from build123d import *

# Parameters (mm, degrees)
ESQUISSE5_W        = 4.75
ESQUISSE5_H        = 4.75
BOSS_EXTRU_3_DEPTH = 4
BOSS_EXTRU_4_DEPTH = 4


with BuildPart() as part:
    # Esquisse1 → Révolution1 (revolve)
    with BuildSketch(Plane(origin=(0, 0, 0), x_dir=(1, 0, 0), z_dir=(0, 1, 0))):
        Polygon((0, 0), (0, 4.75), (142, 4.75), (142, 0), (125.25, 0), (117.25, 0), (24.75, 0), (16.75, 0), align=None)
    revolve(axis=Axis((0, 0, -4.75), (1, 0, 0)))

    # Esquisse5 → Boss.-Extru.3 (add)
    with BuildSketch(Plane(origin=(142, 0, 0), x_dir=(0, 0, -1), z_dir=(1, 0, 0))):
        with Locations((4.75, 0)):
            Rectangle(ESQUISSE5_W, ESQUISSE5_H)
    extrude(amount=BOSS_EXTRU_3_DEPTH)

    # Esquisse6 → Boss.-Extru.4 (add)
    with BuildSketch(Plane.ZY):
        Polygon((-4.75, 2.375), (-7.125, 2.375), (-7.125, -2.375), (-2.375, -2.375), (-2.375, 2.375), align=None)
    extrude(amount=BOSS_EXTRU_4_DEPTH)


solid = part.part
CAD build for the part. Positions are in the model's coordinates, mm. A direction names the side the tool comes from. Coordinates: 2 decimals unless noted, no trailing zeros. Loops run counter-clockwise (first coordinate to the right, second up) from the corner with the lowest first, then second, coordinate; pieces in that order, holes last. Notation, with made-up numbers: (89, 62) - (140, 62) arc R21 ccw to (140, 78) - close; hole circle Ø2 at (-35, -38.75). An arc over 180 degrees is marked (long way). Use one line per item in the form item = value. Start each with the question number.
1) Tool access for faces 1 (the face through (144, 0, -7.125)), 2 (the face through (-2, 0, -7.125)), 3 (the face through (-2, 0, -2.375)): list every direction of +Z, -Z, +X, -X, +Y, -Y with a clear straight run to the whole face (end or side of a thin tool).
2) Band-saw the part on A-A (z = -4.75). Give the cut face in (x, y) (3 decimals), and give its area (3 significant figures).
3) Drill centre lines: L1, parallel to X at y = -3.5, z = -3; L2, parallel to Y at x = 121, z = -4.5; L3, parallel to Z at x = 14, y = -0.5. Where is each one in solid material? Low to high. Write a range as from..to.
4) Band-saw the part on C-C (x = 50). Give the cut face in (y, z), and give its area (3 significant figures).
5) Band-saw the part on B-B (y = 0). Give the cut face in (x, z) (3 decimals), and give its area (3 significant figures).
6) Flat gauge pins, fed straight in: pin 1 (2 mm diameter, centred on x = 144, z = -5.5, fed in from +Y) (3 decimals); pin 2 (2 mm diameter, centred on x = -3, z = -4, fed in from -Y) (3 decimals); pin 3 (4.5 mm diameter, centred on x = 143.5, y = 1, fed in from -Z); pin 4 (4.5 mm diameter, centred on x = 145, y = 1, fed in from +Z) (3 decimals). Where does each tip first touch, or does it go through?
Check values:
q1.face_1 = -Z, +X, +Y, -Y
q1.face_2 = -Z, -X, +Y, -Y
q1.face_3 = +Z, -X, +Y, -Y
q2.outline = (-4, -2.375) - (0, -2.375) - (0, -4.75) - (142, -4.75) - (142, -2.375) - (146, -2.375) - (146, 2.375) - (142, 2.375) - (142, 4.75) - (0, 4.75) - (0, 2.375) - (-4, 2.375) - close
q2.area = 1,390 mm2
q3.L1 = 0..142
q3.L2 = -4.74..4.74
q3.L3 = -9.47..-0.03
q4.outline = circle Ø9.5 at (0, -4.75)
q4.area = 70.9 mm2
q5.outline = (-4, -7.125) - (0, -7.125) - (0, -9.5) - (142, -9.5) - (142, -7.125) - (146, -7.125) - (146, -2.375) - (142, -2.375) - (142, 0) - (0, 0) - (0, -2.375) - (-4, -2.375) - close
q5.area = 1,390 mm2
q6.pin_1 = 2.375
q6.pin_2 = -2.375
q6.pin_3 = -9.5
q6.pin_4 = -2.375
